For this review, take the finished solid that the model builds, in its own axes (mm). A direction names the side the tool comes from. Give positions to 0.01 mm unless a question says otherwise; leave off trailing zeros. Write each loop counter-clockwise with the first axis right and the second up, starting at its lowest first coordinate (ties: lowest second). Pieces come first, ordered by that corner, then holes. Notation, with made-up numbers: (50, -33) -> (93, -33) arc R20 ccw to (93, -27) -> close; hole circle Ø2 at (-3, 3). An arc over 180 degrees is marked (long way). Return JSON: item names as keys, results as strings.
from build123d import *

# Parameters (mm, degrees)
BOSS_EXTRUDE1_DEPTH = 1.143
SKETCH2_R           = 2.6162
BOSS_EXTRUDE2_DEPTH = 3.175


with BuildPart() as part:
    # Sketch1 → Boss-Extrude1 (new body)
    with BuildSketch(Plane(origin=(0, 0, 0), x_dir=(1, 0, 0), z_dir=(0, 1, 0))):
        with BuildLine():
            Line((-7.9629, -10.019330915), (-7.9629, -14.7701))
            ThreePointArc((-7.9629, -14.7701), (-7.293346102, -16.386546102), (-5.6769, -17.0561))
            Line((-5.6769, -17.0561), (5.6769, -17.0561))
            ThreePointArc((5.6769, -17.0561), (7.293346102, -16.386546102), (7.9629, -14.7701))
            Line((7.9629, -14.7701), (7.9629, -10.019330915))
            ThreePointArc((7.9629, -10.019330915), (8.553832276, -8.174549356), (10.10666, -7.016470768))
            Line((10.10666, -7.016470768), (17.42186, -4.50429022))
            ThreePointArc((17.42186, -4.50429022), (20.6375, 0), (17.42186, 4.50429022))
            Line((17.42186, 4.50429022), (3.22159376, 9.380935099))
            ThreePointArc((3.22159376, 9.380935099), (1.633084309, 9.783335082), (0, 9.9187))
            ThreePointArc((0, 9.9187), (-1.633084309, 9.783335082), (-3.22159376, 9.380935099))
            Line((-3.22159376, 9.380935099), (-17.42186, 4.50429022))
            ThreePointArc((-17.42186, 4.50429022), (-20.6375, 0), (-17.42186, -4.50429022))
            Line((-17.42186, -4.50429022), (-10.10666, -7.016470768))
            ThreePointArc((-10.10666, -7.016470768), (-8.553832276, -8.174549356), (-7.9629, -10.019330915))
        make_face()
        with BuildLine():
            ThreePointArc((-15.875, 2.6162), (-18.4912, 0), (-15.875, -2.6162))
            ThreePointArc((-15.875, -2.6162), (-13.2588, 0), (-15.875, 2.6162))
        make_face(mode=Mode.SUBTRACT)
        with BuildLine():
            ThreePointArc((6.796505263, -4.818340964), (0, 8.3312), (-6.796505263, -4.818340964))
            ThreePointArc((-6.796505263, -4.818340964), (-6.483218951, -5.44667203), (-6.3754, -6.140446717))
            Line((-6.3754, -6.140446717), (-6.3754, -15.4686))
            Line((-6.3754, -15.4686), (6.3754, -15.4686))
            Line((6.3754, -15.4686), (6.3754, -9.7536))
            Line((6.3754, -9.7536), (6.3754, -6.140446717))
            ThreePointArc((6.3754, -6.140446717), (6.483218951, -5.44667203), (6.796505263, -4.818340964))
        make_face(mode=Mode.SUBTRACT)
        with BuildLine():
            ThreePointArc((15.875, 2.6162), (13.2588, 0), (15.875, -2.6162))
            ThreePointArc((15.875, -2.6162), (18.4912, 0), (15.875, 2.6162))
        make_face(mode=Mode.SUBTRACT)
    extrude(amount=BOSS_EXTRUDE1_DEPTH)

    # Sketch2 → Boss-Extrude2 (add)
    with BuildSketch(Plane(origin=(0, 1.143, 0), x_dir=(1, 0, 0), z_dir=(0, 1, 0))):
        with BuildLine():
            Line((-7.9629, -10.019330915), (-7.9629, -14.7701))
            ThreePointArc((-7.9629, -14.7701), (-7.293346102, -16.386546102), (-5.6769, -17.0561))
            Line((-5.6769, -17.0561), (5.6769, -17.0561))
            ThreePointArc((5.6769, -17.0561), (7.293346102, -16.386546102), (7.9629, -14.7701))
            Line((7.9629, -14.7701), (7.9629, -10.019330915))
            ThreePointArc((7.9629, -10.019330915), (8.553832276, -8.174549356), (10.10666, -7.016470768))
            Line((10.10666, -7.016470768), (17.42186, -4.50429022))
            ThreePointArc((17.42186, -4.50429022), (20.6375, 0), (17.42186, 4.50429022))
            Line((17.42186, 4.50429022), (3.22159376, 9.380935099))
            ThreePointArc((3.22159376, 9.380935099), (0, 9.9187), (-3.22159376, 9.380935099))
            Line((-3.22159376, 9.380935099), (-17.42186, 4.50429022))
            ThreePointArc((-17.42186, 4.50429022), (-20.6375, 0), (-17.42186, -4.50429022))
            Line((-17.42186, -4.50429022), (-10.10666, -7.016470768))
            ThreePointArc((-10.10666, -7.016470768), (-8.553832276, -8.174549356), (-7.9629, -10.019330915))
        make_face()
        with Locations(Location((15.875, 0, 0), (0, 0, 270))):
            Circle(SKETCH2_R, mode=Mode.SUBTRACT)
        with Locations(Location((-15.875, 0, 0), (0, 0, 270))):
            Circle(SKETCH2_R, mode=Mode.SUBTRACT)
    extrude(amount=BOSS_EXTRUDE2_DEPTH)


solid = part.part
1. The part is to be moulded in two halves that separate along Z. For faces 4 (the flat face through (-8, 0, 5)), 5 (the flat face through (-0.1, 0.6, 15.469)), 6 (the cylindrical face through (20.637, 2.129, 0.083)), say which applies: +Z half, -Z half, draft (parallel to the pull), parting line (faces both ways), or undercut.
Results found:
{"face 4": "draft", "face 5": "undercut", "face 6": "parting line"}
2. Add section C-C, the plane y = 2. Count the separate pieces of the cut face and the enclosed holes in it, plus the area to 3 significant figures.
Results found:
{"separate pieces": "1", "enclosed holes": "2", "area": "646 mm²"}
3. Add section A-A, the plane z = 0. State the section outline as (x, y) points.
Results found:
{"outline": "(-20.64, 0) -> (-18.49, 0) -> (-18.49, 4.32) -> (-20.64, 4.32) -> close; (-13.26, 0) -> (-8.33, 0) -> (-8.33, 1.14) -> (8.33, 1.14) -> (8.33, 0) -> (13.26, 0) -> (13.26, 4.32) -> (-13.26, 4.32) -> close; (18.49, 0) -> (20.64, 0) -> (20.64, 4.32) -> (18.49, 4.32) -> close"}
4. Add section B-B, the plane x = -18. State the section outline as (y, z) points, plus the area to 3 significant figures.
Results found:
{"outline": "(0, -4.26) -> (4.32, -4.26) -> (4.32, -1.53) -> (0, -1.53) -> close; (0, 1.53) -> (4.32, 1.53) -> (4.32, 4.26) -> (0, 4.26) -> close", "area": "23.6 mm²"}
5. Add section D-D, the plane z = 7.5. State the section outline as (x, y) points, plus the area to 3 significant figures.
Results found:
{"outline": "(-9.21, 0) -> (-6.38, 0) -> (-6.38, 1.14) -> (6.38, 1.14) -> (6.38, 0) -> (9.21, 0) -> (9.21, 4.32) -> (-9.21, 4.32) -> close", "area": "64.9 mm²"}
6. For pin 1 (8.5 mm diameter, centred on x = -1.5, z = 4, fed in from -Y); pin 2 (2 mm diameter, centred on y = 3, z = -4.5, fed in from +X); pin 3 (2 mm diameter, centred on x = -11.5, y = 0.5, fed in from +Z), all flat-tipped, find the tip position at first contact; note any pin that passes through.
Results found:
{"pin 1": "stops at y = 1.14", "pin 2": "stops at x = 19.1", "pin 3": "stops at z = 6.88"}
7. For faces 1 (the cylindrical face through (6.48, 0.56, 5.46)), 2 (the flat face through (-7.963, 2, 12)), 3 (the cylindrical face through (-18.43, 2.13, -0.57)), list the 3-axis set-ups (+Z, -Z, +X, -X, +Y, -Y) from which the entire face can be reached by the end or side of a thin tool; tool diameter is ignored.
Results found:
{"face 1": "-Y", "face 2": "+Z, -X, +Y, -Y", "face 3": "+Y, -Y"}
8. To check wall thickness, follow probe 1 along X at (y, z) = (2.7, 0); probe 2 along Z at (x, y) = (15.5, 3.1); probe 3 along Y at (x, z) = (0.5, 12.25). State the ranges of each line that lie inside material, in increasing order.
Results found:
{"probe 1": "x = -20.64 to -18.49, -13.26 to 13.26, 18.49 to 20.64", "probe 2": "z = -5.16 to -2.59, 2.59 to 5.16", "probe 3": "y = 1.14 to 4.32"}
